Read the model definition and answer for the solid it produces. Units are mm, in the model's axes. Face numbers are marked on the shaded views. A direction names the side the tool comes from. Give positions to 0.01 mm unless a question says otherwise; leave off trailing zeros. Order: outer loops, then holes, each group sorted by start corner. A loop starts at its lowest first (then second) coordinate and runs counter-clockwise, first axis right, second up. Notation, with made-up numbers: (9, 35.25) - (20, 35.25) arc R25 ccw to (20, 51.25) - close; hole circle Ø5 at (-40, -26.5). An arc over 180 degrees is marked (long way). Return JSON: item names as keys, results as strings.
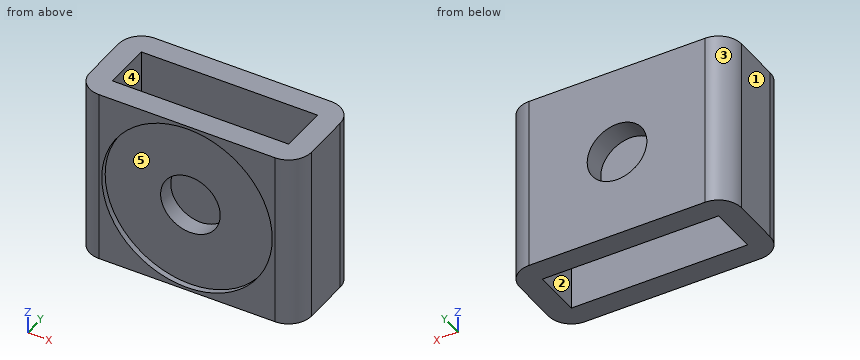
Autodesk Inventor part; units mm, degrees
ref_plane "Work Plane1" through (-9.75, 8.25, 7.75) normal (0, 1, 0) x (1, 0, 0)
ref_plane "YZ Plane" through (0, 0, 0) normal (1, 0, 0) x (0, 1, 0)
ref_plane "XZ Plane" through (0, 0, 0) normal (0, 1, 0) x (-1, 0, 0)
sketch "Sketch1" plane through (0, 0, 0) normal (0, 1, 0) x (-1, 0, 0)
  line L0 (-7.75, -7.75) -> (7.75, -7.75)
  line L1 (7.75, -7.75) -> (7.75, 7.75)
  line L2 (7.75, 7.75) -> (-7.75, 7.75)
  line L3 (-7.75, 7.75) -> (-7.75, -7.75)
  line L4 (-7.75, -7.75) -> (7.75, 7.75) construction
  line L5 (7.75, -7.75) -> (-7.75, 7.75) construction
  line L6 (7.75, 7.75) -> (9.75, 7.75)
  line L7 (9.75, 7.75) -> (9.75, -7.75)
  line L8 (9.75, -7.75) -> (7.75, -7.75)
  line L9 (7.75, -7.75) -> (7.75, 7.75)
  line L10 (-7.75, 7.75) -> (-9.75, 7.75)
  line L11 (-9.75, 7.75) -> (-9.75, -7.75)
  line L12 (-9.75, -7.75) -> (-7.75, -7.75)
  line L13 (-7.75, -7.75) -> (-7.75, 7.75)
  circle A0 centre (0, 0) radius 2.625
  dimension "d0" = 15.5
  dimension "d1" = 15.5
  dimension "d2" = 2
  dimension "d3" = 2
  dimension "d4" = 5.25
extrude "Extrusion1" add sketch "Sketch1" along normal blind 2 contours L3 L2 L1 L0
extrude "Extrusion2" add sketch "Sketch1" along normal blind 8.25 contours L12 L11 L10 L3 | L1 L6 L7 L8
ref_plane "Work Plane1" through (-9.75, 8.25, 7.75) normal (0, 1, 0) x (1, 0, 0)
sketch "Sketch2" plane through (-9.75, 8.25, 7.75) normal (0, 1, 0) x (1, 0, 0)
  line L0 (0, 0) -> (2, 0)
  line L1 (19.5, 15.5) -> (17.5, 15.5)
  line L2 (0, 0) -> (19.5, 0)
  line L3 (19.5, 0) -> (19.5, 15.5)
  line L4 (19.5, 15.5) -> (0, 15.5)
  line L5 (0, 15.5) -> (0, 0)
  circle A0 centre (9.75, 7.75) radius 2.625
  line L6 (17.5, 15.5) -> (2, 15.5)
  line L7 (0, 0) -> (2, 0)
  line L8 (2, 0) -> (2, 15.5)
  line L9 (2, 15.5) -> (0, 15.5)
  line L10 (0, 15.5) -> (0, 0)
  line L11 (17.5, 0) -> (17.5, 15.5)
  line L12 (19.5, 15.5) -> (17.5, 15.5)
  line L13 (17.5, 15.5) -> (17.5, 0)
  line L14 (17.5, 0) -> (19.5, 0)
  line L15 (19.5, 0) -> (19.5, 15.5)
  dimension "d9" = 5.25
extrude "Extrusion3" add sketch "Sketch2" against normal blind 2 contours L8 L4 L11 L2
sketch "Sketch3" plane through (0, 0, 0) normal (0, -1, 0) x (1, 0, 0)
  circle A0 centre (0, 0) radius 7.5
  dimension "d13" = 15
extrude "Extrusion4" cut sketch "Sketch3" against normal blind 0.5
fillet "Fillet2" radius 2 4 edges at (9.75, 8.25, 0) (-9.75, 8.25, 0) (9.75, 0, 0) (-9.75, 0, 0)
Q1. A cutting plane is placed at C-C (x = 0). Write down the section's boundary in (y, z) (3 decimals).
Values:
{"outline": "(0, -7.75) - (2, -7.75) - (2, -2.625) - (0.5, -2.625) - (0.5, -7.5) - (0, -7.5) - close; (0, 7.5) - (0.5, 7.5) - (0.5, 2.625) - (2, 2.625) - (2, 7.75) - (0, 7.75) - close; (6.25, -7.75) - (8.25, -7.75) - (8.25, -2.625) - (6.25, -2.625) - close; (6.25, 2.625) - (8.25, 2.625) - (8.25, 7.75) - (6.25, 7.75) - close"}
Q2. Consider L1, parallel to Z at x = 0, y = 6.8 (3 decimals); L2, parallel to Y at x = -4.5, z = 3; L3, parallel to X at y = 3, z = -7. Determine where each line is inside the solid, lowest interval first.
Values:
{"L1": "z = -7.75 to -2.625, 2.625 to 7.75", "L2": "y = 0.5 to 2, 6.25 to 8.25", "L3": "x = -9.75 to -7.75, 7.75 to 9.75"}
Q3. A cutting plane is placed at D-D (y = 7.25). Write down the section's boundary in (x, z) (3 decimals), and give its area (3 significant figures).
Values:
{"outline": "(-9.482, -7.75) - (9.482, -7.75) - (9.482, 7.75) - (-9.482, 7.75) - close; hole circle Ø5.25 at (0, 0)", "area": "272 mm²"}
Q4. A cutting plane is placed at A-A (z = 0). Write down the section's boundary in (x, y) (3 decimals), and give its area (3 significant figures).
Values:
{"outline": "(-9.75, 2) arc R2 ccw to (-7.75, 0) - (-7.5, 0) - (-7.5, 0.5) - (-2.625, 0.5) - (-2.625, 2) - (-7.75, 2) - (-7.75, 6.25) - (-2.625, 6.25) - (-2.625, 8.25) - (-7.75, 8.25) arc R2 ccw to (-9.75, 6.25) - close; (2.625, 0.5) - (7.5, 0.5) - (7.5, 0) - (7.75, 0) arc R2 ccw to (9.75, 2) - (9.75, 6.25) arc R2 ccw to (7.75, 8.25) - (2.625, 8.25) - (2.625, 6.25) - (7.75, 6.25) - (7.75, 2) - (2.625, 2) - close", "area": "65.7 mm²"}
Q5. For the marked faces 1 and 2, determine the directions among +Z, -Z, +X, -X, +Y, -Y from which every point of the face is accessible in a straight line to the end or side of a thin tool.
Values:
{"face 1": "+Z, -Z, -X, +Y, -Y", "face 2": "+Z, -Z"}
Q6. A cutting plane is placed at B-B (z = -6). Write down the section's boundary in (x, y).
Values:
{"outline": "(-9.75, 2) arc R2 ccw to (-7.75, 0) - (-4.5, 0) - (-4.5, 0.5) - (4.5, 0.5) - (4.5, 0) - (7.75, 0) arc R2 ccw to (9.75, 2) - (9.75, 6.25) arc R2 ccw to (7.75, 8.25) - (-7.75, 8.25) arc R2 ccw to (-9.75, 6.25) - close; hole (-7.75, 2) - (7.75, 2) - (7.75, 6.25) - (-7.75, 6.25) - close"}
Q7. Given pin 1 (4.5 mm diameter, centred on x = 0, z = 0, fed in from -Y), flat-ended and moving along its own axis, determine where the tip first touches the part or whether it passes through.
Values:
{"pin 1": "passes through"}
Q8. Determine the mould class of the marked faces 3, 4 and 5 for opening direction Y: released by +Y, released by -Y, zero draft, split by the parting line, or undercut.
Values:
{"face 3": "released by +Y", "face 4": "undercut", "face 5": "released by -Y"}
